Autodesk Inventor part; units mm, degrees
ref_plane "YZ Plane" through (0, 0, 0) normal (1, 0, 0) x (0, 1, 0)
ref_plane "XZ Plane" through (0, 0, 0) normal (0, 1, 0) x (-1, 0, 0)
ref_plane "XY Plane" through (0, 0, 0) normal (0, 0, 1) x (1, 0, 0)
sketch "Sketch1" plane through (0, 0, 0) normal (0, 1, 0) x (-1, 0, 0)
  line L0 (0, 0) -> (130, 0)
  line L1 (130, 0) -> (130, -40)
  line L2 (130, -40) -> (0, -40)
  line L3 (0, -40) -> (0, 0)
  dimension "d0" = 130
  dimension "d1" = 40
extrude "Extrusion1" add sketch "Sketch1" along normal blind 50
sketch "Sketch3" plane through (-130, 0, 0) normal (0, 0, 1) x (1, 0, 0)
  line L0 (130, 0) -> (0, 0)
  line L1 (0, 0) -> (8, 0)
  line L2 (8, 0) -> (8, 42)
  line L3 (130, 50) -> (0, 50)
  line L4 (122, 0) -> (122, 42)
  line L5 (8, 42) -> (122, 42)
  line L6 (8, 0) -> (122, 0)
  dimension "d8" = 8
  dimension "d9" = 42
extrude "Extrusion3" cut sketch "Sketch3" against normal through all
sketch "Sketch4" plane through (0, 0, 0) normal (0, -1, 0) x (1, 0, 0)
  line L0 (-130, -40) -> (-130, 0)
  line L1 (-8, -40) -> (-122, -40)
  line L2 (-130, 0) -> (-122, 0)
  line L3 (-122, 0) -> (-122, -40)
  line L4 (-122, -40) -> (-130, -40)
  line L5 (-130, -40) -> (-130, 0)
  line L6 (-8, 0) -> (0, 0)
  line L7 (0, 0) -> (0, -40)
  line L8 (0, -40) -> (-8, -40)
  line L9 (-8, -40) -> (-8, 0)
extrude "Extrusion4" add sketch "Sketch4" along normal blind 18
sketch "Sketch7" plane through (-130, 50, -40) normal (-1, 0, 0) x (0, 0, 1)
  line L0 (40, -68) -> (0, -68)
  line L1 (20, -68) -> (20, -50)
  circle A0 centre (20, -46) radius 1.75
  circle A1 centre (16, -50) radius 1.75
  circle A2 centre (20, -54) radius 1.75
  circle A3 centre (24, -50) radius 1.75
  point P0 (40, -50)
  dimension "d23" = 18
  dimension "d25" = 3.5
  dimension "d28" = 360
extrude "Extrusion6" cut sketch "Sketch7" against normal up to surface (8 mm away)
fillet "Fillet1" radius 18.75 4 edges at (-126, -18, -40) (-126, -18, 0) (-4, -18, 0) (-4, -18, -40)
sketch "Sketch8" plane through (0, 50, 0) normal (1, 0, 0) x (0, 0, -1)
  line L0 (16, -50) -> (24, -50)
  line L1 (20, -54) -> (20, -46)
  circle A0 centre (20, -50) radius 6.4
  point P0 (0, -50)
  dimension "d33" = 12.8
extrude "Extrusion7" add sketch "Sketch8" against normal blind 15
sketch "Sketch9" plane through (-122, 42, 0) normal (0, -1, 0) x (1, 0, 0)
  line L0 (-8, 0) -> (122, 0)
  line L1 (122, -40) -> (-8, -40)
  circle A0 centre (77, -10) radius 2
  circle A1 centre (77, -30) radius 2
  circle A2 centre (37, -30) radius 2
  circle A3 centre (37, -10) radius 2
  dimension "d40" = 4
extrude "Extrusion8" cut sketch "Sketch9" against normal through all
properties part number "tilt_output_bracket"
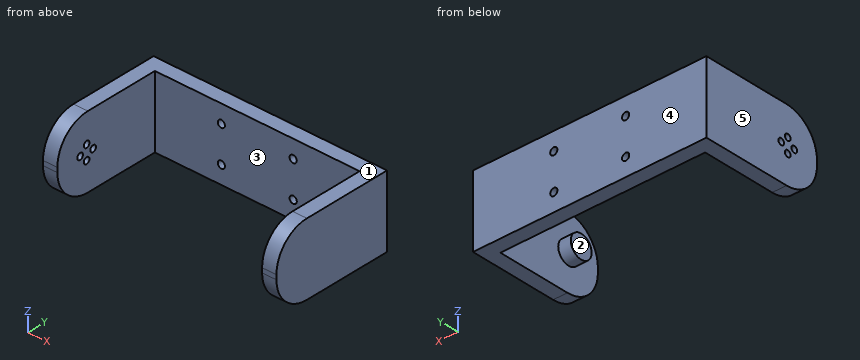
Input: part model. Units: mm. Frame: model coordinates. Face numbers are marked on the shaded views. A direction names the side the tool comes from. Round coordinates to 2 decimals unless told otherwise and drop trailing zeros. Loops run counter-clockwise (first coordinate to the right, second up) from the corner with the lowest first, then second, coordinate; pieces in that order, holes last. Notation, with made-up numbers: (-9.5, -35.75) -> (10.5, -35.75) arc R21 ccw to (10.5, -7.75) -> close; hole circle Ø5 at (-13, 83). An arc over 180 degrees is marked (long way). Write each question's results on one line, items separated by ' | '.
1. Section B-B (x = -85). Return loops of the section in (y, z).
Geometry results:
outline: (42, -40) -> (50, -40) -> (50, -32) -> (42, -32) -> close; (42, -28) -> (50, -28) -> (50, -12) -> (42, -12) -> close; (42, -8) -> (50, -8) -> (50, 0) -> (42, 0) -> close
2. Set-up query: the marked faces 1 and 2. Return all of +Z, -Z, +X, -X, +Y, -Y with unobstructed straight access to the full face (end or side cutting, diameter ignored); none if empty.
Geometry results:
face 1: +Z, +X, -X, +Y, -Y | face 2: +Z, -Z, -Y
3. First-contact query: P1, Ø5, axis at x = -85, z = -30, coming from the -Y side. Flat tip, straight axial feed; report the tip coordinate or a pass-through.
Geometry results:
P1: y = 42
4. Section D-D (z = -10). Return loops of the section in (x, y), and give its area (3 significant figures).
Geometry results:
outline: (-130, -15.83) -> (-122, -15.83) -> (-122, 42) -> (-87, 42) -> (-87, 50) -> (-130, 50) -> close; (-83, 42) -> (-47, 42) -> (-47, 50) -> (-83, 50) -> close; (-43, 42) -> (-8, 42) -> (-8, -15.83) -> (0, -15.83) -> (0, 50) -> (-43, 50) -> close | area: 1,900 mm2
5. Mould query, pull axis X, two halves, no side actions, for the marked faces 3, 4 and 5. Classes: +X half, -X half, draft (parallel to the pull), parting line (faces both ways), or undercut.
Geometry results:
face 3: undercut | face 4: draft | face 5: -X half
6. Ray query, line 1 (Y direction, x = -124, z = -20); line 2 (Z direction, x = -85, y = 46); line 3 (X direction, y = -6.5, z = -5.5). Return the intervals inside material, ascending. Write a range as from..to.
Geometry results:
line 1: -18..-5.75, -2.25..2.25, 5.75..50 | line 2: -40..-32, -28..-12, -8..0 | line 3: -130..-122, -8..0
7. Section C-C (z = -16). Return loops of the section in (x, y).
Geometry results:
outline: (-130, -17.8) -> (-122, -17.8) -> (-122, -1.75) -> (-130, -1.75) -> close; (-130, 1.75) -> (-122, 1.75) -> (-122, 42) -> (-8, 42) -> (-8, 5) -> (-15, 5) -> (-15, -5) -> (-8, -5) -> (-8, -17.8) -> (0, -17.8) -> (0, 50) -> (-130, 50) -> close
8. Section A-A (y = 8). Return loops of the section in (x, z), and give its area (3 significant figures).
Geometry results:
outline: (-130, -40) -> (-122, -40) -> (-122, 0) -> (-130, 0) -> close; (-8, -40) -> (0, -40) -> (0, 0) -> (-8, 0) -> close | area: 640 mm2
